Can you work these out from the model? Positions are in its coordinate system, mm. A direction names the side the tool comes from. Give positions to 0.01 mm unless a question says otherwise; leave off trailing zeros. Write each loop counter-clockwise with the first axis right and the second up, starting at its lowest first coordinate (ties: lowest second). Pieces come first, ordered by that corner, then holes. Notation, with made-up numbers: M 34.25,74 L 80.25,74 A14 cw 80.25,97 Z; hole C 83.5,-32 d6. An arc over 180 degrees is marked long. Use CSV: the item, a comma, the result in double quotes. Start each with the question number.
from build123d import *

# Parameters (mm, degrees)
SKIZZE1_W                       = 1400
SKIZZE1_H                       = 680
AUFSATZ_LINEAR_AUSTRAGEN1_DEPTH = 40
SKIZZE2_W                       = 35
SKIZZE2_H                       = 35
AUFSATZ_LINEAR_AUSTRAGEN2_DEPTH = 710
SKIZZE3_W                       = 1365
SKIZZE3_H                       = 645
AUFSATZ_LINEAR_AUSTRAGEN3_DEPTH = 450


with BuildPart() as part:
    # Skizze1 → Aufsatz-Linear austragen1 (new body)
    with BuildSketch(Plane.XY):
        with Locations((679.568580104, -330.209944633)):
            Rectangle(SKIZZE1_W, SKIZZE1_H)
    extrude(amount=AUFSATZ_LINEAR_AUSTRAGEN1_DEPTH)

    # Skizze2 → Aufsatz-Linear austragen2 (add)
    with BuildSketch(Plane(origin=(0, 0, 0), x_dir=(-1, 0, 0), z_dir=(0, 0, -1))):
        with Locations((-1362.068580104, -7.709944633)):
            Rectangle(SKIZZE2_W, SKIZZE2_H)
        with Locations((-1362.068580104, -652.709944633)):
            Rectangle(SKIZZE2_W, SKIZZE2_H)
        with Locations((2.931419896, -7.709944633)):
            Rectangle(SKIZZE2_W, SKIZZE2_H)
        with Locations((2.931419896, -652.709944633)):
            Rectangle(SKIZZE2_W, SKIZZE2_H)
    extrude(amount=AUFSATZ_LINEAR_AUSTRAGEN2_DEPTH)

    # Skizze3 → Aufsatz-Linear austragen3 (add)
    with BuildSketch(Plane(origin=(0, 0, 0), x_dir=(-1, 0, 0), z_dir=(0, 0, -1))):
        with Locations((-679.568580104, -330.209944633)):
            Rectangle(SKIZZE3_W, SKIZZE3_H)
    extrude(amount=AUFSATZ_LINEAR_AUSTRAGEN3_DEPTH)


solid = part.part
(1) Please list where these lines run through material, in increasing order: L1, parallel to Z at x = 644, y = -43; L2, parallel to Y at x = 1172, z = -240; L3, parallel to X at y = -221, z = -421.5. Write a range as [from, to].
(2) Thinking about a two-plate mould opening in Y: for faces 5 (the face through (683, 9.79, 28)), 6 (the face through (-20.431, -332, 24)), 7 (the face through (-7, -635.21, -429)), 8 (the face through (1366, -635.21, -429)), which applies, released by +Y, released by -Y, zero draft, split by the parting line, or undercut?
(3) Which directions (+Z, -Z, +X, -X, +Y, -Y) give clear straight access to the entire face, cutting with the end or side of a thin tool? Please do faces 1 (the face through (-2.931, -334, -222)), 2 (the face through (689, -652.71, -222)), 3 (the face through (1362.069, -334, -222)), 4 (the face through (689, -7.71, -222)).
(4) I want a section at D-D (z = -318.5). Write out the boundary of the cut face in (x, y).
(5) I want a section at B-B (x = 605). Write out the boundary of the cut face in (y, z).
(6) Will these pins go through, and if not, where does the flat tip stop? pin 1 Ø5 at (y, z) = (-201, -444.5) entering from -X; pin 2 Ø4 at (x, z) = (219.5, -402.5) entering from -Y; pin 3 Ø2 at (x, z) = (262, -176.5) entering from +Y.
(7) I want a section at C-C (y = -301). Write out the boundary of the cut face in (x, z).
(8) I want a section at A-A (z = -609.5). Write out the boundary of the cut face in (x, y), and give its area (3 significant figures).
Geometry results:
1,L1,"z = [-450, 40]"
1,L2,"y = [-652.71, -7.71]"
1,L3,"x = [-2.93, 1362.07]"
2,face 5,"released by +Y"
2,face 6,"zero draft"
2,face 7,"undercut"
2,face 8,"undercut"
3,face 1,"-Z, -X"
3,face 2,"-Z, -Y"
3,face 3,"-Z, +X"
3,face 4,"-Z, +Y"
4,outline,"M -20.43,-670.21 L 14.57,-670.21 L 14.57,-652.71 L 1344.57,-652.71 L 1344.57,-670.21 L 1379.57,-670.21 L 1379.57,-635.21 L 1362.07,-635.21 L 1362.07,-25.21 L 1379.57,-25.21 L 1379.57,9.79 L 1344.57,9.79 L 1344.57,-7.71 L 14.57,-7.71 L 14.57,9.79 L -20.43,9.79 L -20.43,-25.21 L -2.93,-25.21 L -2.93,-635.21 L -20.43,-635.21 Z"
5,outline,"M -670.21,0 L -652.71,0 L -652.71,-450 L -7.71,-450 L -7.71,0 L 9.79,0 L 9.79,40 L -670.21,40 Z"
6,pin 1,"stops at x = -2.93"
6,pin 2,"stops at y = -652.71"
6,pin 3,"stops at y = -7.71"
7,outline,"M -20.43,0 L -2.93,0 L -2.93,-450 L 1362.07,-450 L 1362.07,0 L 1379.57,0 L 1379.57,40 L -20.43,40 Z"
8,outline,"M -20.43,-670.21 L 14.57,-670.21 L 14.57,-635.21 L -20.43,-635.21 Z; M -20.43,-25.21 L 14.57,-25.21 L 14.57,9.79 L -20.43,9.79 Z; M 1344.57,-670.21 L 1379.57,-670.21 L 1379.57,-635.21 L 1344.57,-635.21 Z; M 1344.57,-25.21 L 1379.57,-25.21 L 1379.57,9.79 L 1344.57,9.79 Z"
8,area,"4,900 mm2"
